Can you work these out from the model? Positions are in its coordinate system, mm. Face numbers are marked on the shaded views. A direction names the side the tool comes from. Give positions to 0.01 mm unless a question says otherwise; leave off trailing zeros. Order: outer loops, then holes, each group sorted by start corner. A loop starts at its lowest first (then second) coordinate and runs counter-clockwise, first axis right, second up. Notation, with made-up numbers: M 73,21.25 L 100,21.25 A7 cw 100,30.25 Z; hole C 63,7.25 d2. An arc over 180 degrees is marked long. Use a Markdown table: item, result. Add a question column.
from build123d import *
from build123d.topology import SkipClean

# Parameters (mm, degrees)
SKETCH2_R           = 9.5
SKETCH2_R_2         = 17.5
BOSS_EXTRUDE1_DEPTH = 36
CUT_EXTRUDE1_DEPTH  = 12
CUT_EXTRUDE2_DEPTH  = 12
SKETCH6_R           = 16
SKETCH6_R_2         = 9.5
CUT_EXTRUDE3_DEPTH  = 5.5
SKETCH7_R           = 16
SKETCH7_R_2         = 9.5
CUT_EXTRUDE4_DEPTH  = 5.5
SKETCH8_R           = 24
SKETCH8_R_2         = 17.5
BOSS_EXTRUDE2_DEPTH = 36
SKETCH9_R           = 16
SKETCH9_R_2         = 9.5
BOSS_EXTRUDE4_DEPTH = 25


with BuildPart() as part:
    # Sketch2 → Boss-Extrude1 (new body)
    with BuildSketch(Plane.XY):
        with BuildLine():
            ThreePointArc((10.583005244, 12), (-15.998110701, 0.245873959), (10.209239534, -12.319554705))
            Line((10.209239534, -12.319554705), (10.526232528, -12.049831068))
            ThreePointArc((10.526232528, -12.049831068), (10.554648294, -12.024949039), (10.583005244, -12))
            Line((10.583005244, -12), (104.215390309, -12))
            ThreePointArc((104.215390309, -12), (149, 0), (104.215390309, 12))
            Line((104.215390309, 12), (10.583005244, 12))
        make_face()
        Circle(SKETCH2_R, mode=Mode.SUBTRACT)
        with Locations((125, 0)):
            Circle(SKETCH2_R_2, mode=Mode.SUBTRACT)
    extrude(amount=BOSS_EXTRUDE1_DEPTH)

    # Sketch3 → Cut-Extrude1 (cut)
    with BuildSketch(Plane(origin=(0, 0, 0), x_dir=(-1, 0, 0), z_dir=(0, 0, -1))):
        with BuildLine():
            Line((-104.215390309, 12), (-10.583005244, 12))
            ThreePointArc((-10.583005244, 12), (-15.553567993, 0), (-10.583005244, -12))
            Line((-10.583005244, -12), (-104.215390309, -12))
            ThreePointArc((-104.215390309, -12), (-101.138897743, 0), (-104.215390309, 12))
        make_face()
    extrude(amount=-CUT_EXTRUDE1_DEPTH, mode=Mode.SUBTRACT)

    # Sketch4 → Cut-Extrude2 (cut)
    with BuildSketch(Plane.XY.offset(36)):
        with BuildLine():
            Line((10.583005244, 12), (104.215390309, 12))
            ThreePointArc((104.215390309, 12), (101, 0), (104.215390309, -12))
            Line((104.215390309, -12), (10.367736031, -12.184692887))
            ThreePointArc((10.367736031, -12.184692887), (15.484184535, -0.136930157), (10.583005244, 12))
        make_face()
    extrude(amount=-CUT_EXTRUDE2_DEPTH, mode=Mode.SUBTRACT)

    # Sketch6 → Cut-Extrude3 (cut)
    with BuildSketch(Plane.XY.offset(36)):
        Circle(SKETCH6_R)
        Circle(SKETCH6_R_2, mode=Mode.SUBTRACT)
    extrude(amount=-CUT_EXTRUDE3_DEPTH, mode=Mode.SUBTRACT)

    # Sketch7 → Cut-Extrude4 (cut)
    with BuildSketch(Plane(origin=(0, 0, 0), x_dir=(-1, 0, 0), z_dir=(0, 0, -1))):
        Circle(SKETCH7_R)
        Circle(SKETCH7_R_2, mode=Mode.SUBTRACT)
    extrude(amount=-CUT_EXTRUDE4_DEPTH, mode=Mode.SUBTRACT)

    # Sketch8 → Boss-Extrude2 (add)
    with BuildSketch(Plane(origin=(0, 0, 0), x_dir=(-1, 0, 0), z_dir=(0, 0, -1))):
        with Locations(Location((-125, 0, 0), (0, 0, 180))):
            Circle(SKETCH8_R)
        with Locations(Location((-125, 0, 0), (0, 0, 180))):
            Circle(SKETCH8_R_2, mode=Mode.SUBTRACT)
    extrude(amount=-BOSS_EXTRUDE2_DEPTH)

    # Sketch9 → Boss-Extrude4 (add)
    with SkipClean():  # the faces are left unmerged after this step: merging them gives an invalid solid
        with BuildSketch(Plane(origin=(0, 0, 5.5), x_dir=(-1, 0, 0), z_dir=(0, 0, -1))):
            with Locations(Location((0, 0, 0), (0, 0, 230.351389725))):
                Circle(SKETCH9_R)
            Circle(SKETCH9_R_2, mode=Mode.SUBTRACT)
        extrude(amount=-BOSS_EXTRUDE4_DEPTH)


solid = part.part
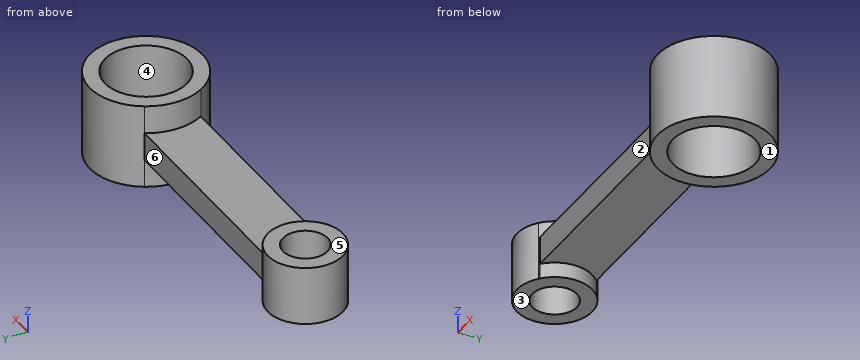
1. On a 3-axis mill with a long thin cutter (end or side, diameter ignored), from which of +Z, -Z, +X, -X, +Y, -Y can I reach the whole of each face in a straight line? I mean the marked faces 1, 2 and 3. Say none if no direction works.
2. Will these pins go through, and if not, where does the flat tip stop? pin 1 (12 mm diameter, centred on x = 56, z = 11.5, fed in from -Y); pin 2 (19 mm diameter, centred on x = 40, y = 1.5, fed in from +Z); pin 3 (1.5 mm diameter, centred on y = 4.5, z = 23, fed in from +X); pin 4 (21 mm diameter, centred on x = 125, y = 0, fed in from +Z).
3. If we section it at A-A, the plane y = 0: List the corners of the cut face in (x, z) for me.
4. If we section it at C-C, the plane z = 15: List the corners of the cut face in (x, y) for me, then the cut area to 3 significant figures.
5. If we section it at B-B, the plane x = 125: List the corners of the cut face in (y, z) for me, then the cut area to 3 significant figures.
6. We'd pull the mould along Y, two halves only. Please class the marked faces 4, 5 and 6: +Y half, -Y half, draft (parallel to the pull), parting line (faces both ways), or undercut.
7. If we section it at D-D, the plane x = 0: List the corners of the cut face in (y, z) for me, then the cut area to 3 significant figures.
8. I need wall thicknesses on L1, parallel to Y at x = 125, z = 13; L2, parallel to Y at x = 0, z = 22.75; L3, parallel to X at y = -5, z = 11.5. Which ranges of each line are inside material? Lowest first, please. Write a range as [from, to].
Geometry results:
| question | item | result |
|---|---|---|
| 1 | face 1 | -Z, +X, -X, +Y, -Y |
| 1 | face 2 | +Z, -Z, -Y |
| 1 | face 3 | -Z, -X, +Y, -Y |
| 2 | pin 1 | stops at y = -12 |
| 2 | pin 2 | stops at z = 24 |
| 2 | pin 3 | stops at x = 148.71 |
| 2 | pin 4 | passes through |
| 3 | outline | M -16,5.5 L -9.5,5.5 L -9.5,30.5 L -16,30.5 Z; M 9.5,5.5 L 16,5.5 L 16,12 L 101,12 L 101,0 L 107.5,0 L 107.5,36 L 101,36 L 101,24 L 16,24 L 16,30.5 L 9.5,30.5 Z; M 142.5,0 L 149,0 L 149,36 L 142.5,36 Z |
| 4 | outline | M 10.53,-12.05 A16 ccw 10.58,-12 L 104.22,-12 A24 ccw long 104.22,12 L 10.58,12 A16 ccw long Z; hole C 0,0 d19; hole C 125,0 d35 |
| 4 | area | 3,470 mm^2 |
| 5 | outline | M -24,0 L -17.5,0 L -17.5,36 L -24,36 Z; M 17.5,0 L 24,0 L 24,36 L 17.5,36 Z |
| 5 | area | 468 mm^2 |
| 6 | face 4 | undercut |
| 6 | face 5 | draft |
| 6 | face 6 | +Y half |
| 7 | outline | M -16,5.5 L -9.5,5.5 L -9.5,30.5 L -16,30.5 Z; M 9.5,5.5 L 16,5.5 L 16,30.5 L 9.5,30.5 Z |
| 7 | area | 325 mm^2 |
| 8 | L1 | y = [-24, -17.5], [17.5, 24] |
| 8 | L2 | y = [-16, -9.5], [9.5, 16] |
| 8 | L3 | x = [-15.2, -8.08], [8.08, 15.2], [101.53, 108.23], [141.77, 148.47] |
